from build123d import *

# Parameters (mm, degrees)
SKETCH_1_W           = 23.8
SKETCH_1_H           = 9.7
SKETCH_1_W_2         = 22
SKETCH_1_H_2         = 7.9
EXTRUDE_1_DEPTH      = 93.5
SKETCH_5_W           = 30.862098313
SKETCH_5_H           = 22
CUT_EXTRUDE_1_DEPTH  = 5
EXTRUDE_3_DEPTH      = 3
EXTRUDE_3_DEPTH_BACK = 2.5
CUT_EXTRUDE_2_DEPTH  = 2.3
CUT_EXTRUDE_3_DEPTH  = 2.3
SKETCH_10_W          = 27.414514358
SKETCH_10_H          = 5.206733811
EXTRUDE_4_DEPTH      = 5.45
EXTRUDE_5_DEPTH      = 23.8
CUT_EXTRUDE_4_DEPTH  = 10
CUT_EXTRUDE_5_DEPTH  = 5
FILLET_2_R           = 0.7


with BuildPart() as part:
    # 草图1 → 凸台-拉伸1 (new body)
    with BuildSketch(Plane(origin=(0, 0, 0), x_dir=(0, 0, -1), z_dir=(1, 0, 0))):
        Rectangle(SKETCH_1_W, SKETCH_1_H)
        Rectangle(SKETCH_1_W_2, SKETCH_1_H_2, mode=Mode.SUBTRACT)
    extrude(amount=EXTRUDE_1_DEPTH)

    # 草图5 → 切除-拉伸1 (cut)
    with BuildSketch(Plane(origin=(0, 4.85, 0), x_dir=(1, 0, 0), z_dir=(0, 1, 0))):
        with Locations((12.679771903, 0)):
            Rectangle(SKETCH_5_W, SKETCH_5_H)
    extrude(amount=-CUT_EXTRUDE_1_DEPTH, mode=Mode.SUBTRACT)

    # 草图7 → 凸台-拉伸3 (add, two sides: drawn at the far end of the back side and taken through both)
    with BuildSketch(Plane.ZY.offset(-EXTRUDE_3_DEPTH_BACK)):
        Polygon((-11, 4.85), (11, 4.85), (11.9, 4.85), (11.9, -4.85), (-11.9, -4.85), (-11.9, 4.85), align=None)
    extrude(amount=EXTRUDE_3_DEPTH + EXTRUDE_3_DEPTH_BACK)

    # 草图8 → 切除-拉伸2 (cut)
    with BuildSketch(Plane.XY.offset(11.9)):
        Polygon((0.878787233, 4.85), (1.766547003, 2.85), (21.968929262, 2.85), (21.968929262, 4.85), align=None)
    extrude(amount=-CUT_EXTRUDE_2_DEPTH, mode=Mode.SUBTRACT)

    # 草图9 → 切除-拉伸3 (cut)
    with BuildSketch(Plane(origin=(0, 0, -11.9), x_dir=(-1, 0, 0), z_dir=(0, 0, -1))):
        with BuildLine():
            Line((2.347261018, 3.516538115), (3, 3.516538115))
            Line((3, 3.516538115), (3, 4.85))
            Line((3, 4.85), (0.483692493, 4.85))
            add(Edge.make_bspline(
                [(0.483692493, 4.85), (1.57048018, 4.409488755), (2.347261018, 3.516538115)],
                knots=[0, 0, 0, 1, 1, 1], degree=2))
        make_face()
    extrude(amount=-CUT_EXTRUDE_3_DEPTH, mode=Mode.SUBTRACT)

    # 草图10 → 凸台-拉伸4 (add)
    with BuildSketch(Plane.XY.offset(11.9)):
        with Locations((17.041287755, 0.106962124)):
            Rectangle(SKETCH_10_W, SKETCH_10_H)
    extrude(amount=EXTRUDE_4_DEPTH)

    # 草图11 → 凸台-拉伸5 (add)
    with BuildSketch(Plane(origin=(0, 0, -11.9), x_dir=(-1, 0, 0), z_dir=(0, 0, -1))):
        Polygon((-93.5, -4.85), (-93.5, -5.65), (-92.9, -5.65), (-91.3, -4.85), align=None)
        Polygon((-91.3, 4.85), (-92.8, 5.85), (-93.5, 5.85), (-93.5, 4.85), align=None)
    extrude(amount=-EXTRUDE_5_DEPTH)

    # 草图12 → 切除-拉伸4 (cut)
    with BuildSketch(Plane(origin=(0, 2.71032903, 0), x_dir=(1, 0, 0), z_dir=(0, 1, 0))):
        with BuildLine():
            Line((30.354179143, -13.864715533), (30.354179143, -11.9))
            Line((30.354179143, -11.9), (31.029316872, -11.9))
            Line((31.029316872, -11.9), (31.273931991, -17.729634416))
            Line((31.273931991, -17.729634416), (25.559722807, -17.35))
            add(Edge.make_bspline(
                [(25.559722807, -17.35), (28.738846795, -16.858311071), (30.354179143, -13.864715533)],
                knots=[0, 0, 0, 1, 1, 1], degree=2))
        make_face()
        Polygon((11.717782686, -17.35), (11.717782686, -11.9), (1.430390108, -11.9), (1.430390108, -18.181001755), align=None)
    extrude(amount=-CUT_EXTRUDE_4_DEPTH, mode=Mode.SUBTRACT)

    # 草图14 → 切除-拉伸5 (cut)
    with BuildSketch(Plane(origin=(93.5, 0, 0), x_dir=(0, 0, -1), z_dir=(1, 0, 0))):
        Polygon((-11, 5.85), (-11.9, 5.85), (-11.9, 4.85), (-11, 4.85), (-11, -4.85), (-11.9, -4.85), (-11.9, -5.65), (-11, -5.65), (-10.4, -5.65), (-10.4, 5.85), align=None)
        Polygon((11.9, 5.85), (11, 5.85), (10.4, 5.85), (10.4, -5.65), (11, -5.65), (11.9, -5.65), (11.9, -4.85), (11, -4.85), (11, 4.85), (11.9, 4.85), align=None)
    extrude(amount=-CUT_EXTRUDE_5_DEPTH, mode=Mode.SUBTRACT)

    # 圆角2
    fillet_2_edges = [part.edges().sort_by_distance(p)[0] for p in [
        (46.508153753, 4.85, -11.9),
        (45.25, -4.85, -11.9),
        (45.25, -4.85, 11.9),
        (57.734464631, 4.85, 11.9),
    ]]
    fillet(fillet_2_edges, radius=FILLET_2_R)


solid = part.part
Model file for the job. Use its own axes, mm. A direction names the side the tool comes from. Round coordinates to 2 decimals unless told otherwise and drop trailing zeros. Order: outer loops, then holes, each group sorted by start corner. A loop starts at its lowest first (then second) coordinate and runs counter-clockwise, first axis right, second up.
(1) Pin check, flat tips, straight feed: pin 1 (8 mm diameter, centred on x = 66.5, z = 7.5, fed in from -Y); pin 2 (6 mm diameter, centred on y = 3, z = 1.5, fed in from +X); pin 3 (3 mm diameter, centred on x = 23.5, z = -3.5, fed in from +Y); pin 4 (0.6 mm diameter, centred on x = 90, y = 5, fed in from +Z). Stop position of each tip, or through.
(2) Band-saw the part on B-B (x = 40.5). List the corners of the cut face in (y, z), then the cut area to 3 significant figures.
(3) Pull direction Z, two halves, no side cores. Call faces 1 (the face through (2, 4, 9.6)), 2 (the face through (2.5, 1, 0)), 3 (the face through (21, 2.71, 15)): released by +Z, released by -Z, zero draft, split by the parting line, or undercut.
(4) Drill centre lines: line 1 (Z direction, x = 23, y = -2.75); line 2 (Y direction, x = 42, z = 4.5); line 3 (X direction, y = 0.75, z = 3). Where is each one in solid material? Low to high.
(5) Band-saw the part on A-A (z = -2.75). List the corners of the cut face in (x, y), then the cut area to 3 significant figures.
(6) 3-axis set-ups, long thin cutter, end or side, ignore diameter. For faces 4 (the face through (60, 3.95, 0)), 5 (the face through (30.354, 0, 13)), 6 (the face through (1.3, 3.9, 10.8)), 7 (the face through (21, -2.496, 15)), 8 (the face through (11.718, 0, 15)): which of +Z, -Z, +X, -X, +Y, -Y reach the whole face in a straight line?
Verdict:
1. pin 1: stops at y = -4.85
1. pin 2: stops at x = 93.5
1. pin 3: stops at y = -3.95
1. pin 4: stops at z = 11.63
2. outline: (-4.85, -11.2) arc R0.7 ccw to (-4.15, -11.9) - (4.15, -11.9) arc R0.7 ccw to (4.85, -11.2) - (4.85, 11.2) arc R0.7 ccw to (4.15, 11.9) - (-4.15, 11.9) arc R0.7 ccw to (-4.85, 11.2) - close; hole (-3.95, -11) - (3.95, -11) - (3.95, 11) - (-3.95, 11) - close
2. area: 56.6 mm2
3. face 1: released by +Z
3. face 2: undercut
3. face 3: zero draft
4. line 1: z = -11.9 to -11, 11 to 11.9
4. line 2: y = -4.85 to -3.95, 3.95 to 4.85
4. line 3: x = -3 to 2.5
5. outline: (-3, -4.85) - (91.3, -4.85) - (92.9, -5.65) - (93.5, -5.65) - (93.5, -3.95) - (2.5, -3.95) - (2.5, 4.85) - (-3, 4.85) - close; (28.11, 3.95) - (93.5, 3.95) - (93.5, 5.85) - (92.8, 5.85) - (91.3, 4.85) - (28.11, 4.85) - close
5. area: 197 mm2
6. face 4: +X
6. face 5: +Z, +X, +Y, -Y
6. face 6: +Z, +Y
6. face 7: +Z, +X, -X, -Y
6. face 8: +Z, -X, +Y, -Y
